Autodesk Inventor part; units mm, degrees
ref_plane "YZ Plane" through (0, 0, 0) normal (1, 0, 0) x (0, 1, 0)
ref_plane "XZ Plane" through (0, 0, 0) normal (0, 1, 0) x (-1, 0, 0)
ref_plane "XY Plane" through (0, 0, 0) normal (0, 0, 1) x (1, 0, 0)
sketch "Sketch1" plane through (0, 0, 0) normal (0, 0, 1) x (1, 0, 0)
  circle A0 centre (0, 0) radius 25.4
  dimension "d0" = 50.8
extrude "Extrusion1" add sketch "Sketch1" along normal blind 25.4 and the other way blind 101.6
sketch "Sketch2" plane through (0, 0, 0) normal (0, 1, 0) x (-1, 0, 0)
  line L0 (0, -25.4) -> (0, 152.4) construction
  line L1 (25.4, 25.4) -> (-25.4, 25.4) construction
  line L2 (0, 25.4) -> (-50.8, 25.4)
  line L3 (-50.8, 25.4) -> (-50.8, 127)
  line L4 (-50.8, 127) -> (0, 127)
  line L5 (0, 127) -> (0, 25.4)
  point P0 (0, 0)
  dimension "d8" = 50.8
  dimension "d9" = 101.6
revolve "Revolution1" add sketch "Sketch2" angle 360 about axis through (0, 0, -10) along (0, 0, 1)
sketch "Sketch3" plane through (0, 0, 0) normal (1, 0, 0) x (0, 1, 0)
  line L0 (50.8, 127) -> (-50.8, 127) construction
  line L1 (31.75, 127) -> (-31.75, 127)
  line L2 (-31.75, 127) -> (-31.75, 50.8)
  line L3 (-31.75, 50.8) -> (31.75, 50.8)
  line L4 (31.75, 50.8) -> (31.75, 127)
  line L5 (0, -25.4) -> (0, 152.4) construction
  point P0 (0, 0)
  point P1 (0, 50.8)
  dimension "d11" = 0
  dimension "d12" = 76.2
  dimension "d13" = 63.5
extrude "Extrusion2" cut sketch "Sketch3" along normal mid plane 254
sketch "Sketch4" plane through (0, 0, 0) normal (0, 1, 0) x (-1, 0, 0)
  line L0 (-39.6557, 127) -> (39.6557, 127) construction
  line L1 (39.6557, 127) -> (39.6557, 50.8) construction
  line L2 (-39.6557, 50.8) -> (-39.6557, 127) construction
  line L3 (-29.4957, 50.8) -> (-29.4957, 94.9643)
  line L4 (39.6557, 50.8) -> (-39.6557, 50.8) construction
  line L5 (29.4957, 94.9643) -> (29.4957, 50.8)
  arc A0 (29.4957, 94.9643) -> (-29.4957, 94.9643) centre (0, 94.9643) ccw
  line L6 (-29.4957, 50.8) -> (-112.68, 50.8)
  line L7 (-112.68, 50.8) -> (-112.68, 137.8838)
  line L8 (-112.68, 137.8838) -> (83.0957, 137.8838)
  line L9 (83.0957, 137.8838) -> (83.0957, 50.8)
  line L10 (83.0957, 50.8) -> (29.4957, 50.8)
  line L11 (39.6557, 127) -> (-39.6557, 127) construction
  point P0 (0, 0)
  point P1 (0, 124.46)
  point P2 (0, 127)
  point P3 (0, 127)
  dimension "d16" = 10.16
  dimension "d17" = 10.16
  dimension "d24" = 2.54
extrude "Extrusion3" cut sketch "Sketch4" along normal mid plane 254
sketch "Sketch5" plane through (0, 31.75, 94.9643) normal (0, -1, 0) x (1, 0, 0)
  circle A0 centre (0, 0) radius 15.875
  line L0 (29.4957, 0) -> (29.4957, -44.1643) construction
  line L1 (-29.4957, 0) -> (29.4957, 0) construction
  point P0 (0, -94.9643)
  dimension "d21" = 31.75
extrude "Extrusion4" add sketch "Sketch5" along normal up to next
properties part number "u_joint"
The listing builds one solid part. Answer for the finished solid, in the listing's coordinates (mm). A direction names the side the tool comes from. Give positions to 0.01 mm unless a question says otherwise; leave off trailing zeros. Write each loop counter-clockwise with the first axis right and the second up, starting at its lowest first coordinate (ties: lowest second). Pieces come first, ordered by that corner, then holes. Notation, with made-up numbers: (21.25, 13) -> (33.25, 13) arc R23 cw to (33.25, 45) -> close; hole circle Ø4 at (-34.75, -2.75). An arc over 180 degrees is marked (long way). Use a Markdown table: item, result.
(1) For faces 5 (the cylindrical face through (-5.506, -24.796, -37.211)), 6 (the flat face through (-7, -31.75, 80)), 7 (the flat face through (-29.496, 36, 73)), 8 (the flat face through (29.496, -37, 73)), determine the directions among +Z, -Z, +X, -X, +Y, -Y from which every point of the face is accessible in a straight line to the end or side of a thin tool.
Return value:
| item | result |
|---|---|
| face 5 | -Z |
| face 6 | none |
| face 7 | +Z, -X, +Y, -Y |
| face 8 | +Z, +X, +Y, -Y |
(2) Determine the mould class of faces 1 (the flat face through (10.6, 23.3, 25.4)), 2 (the cylindrical face through (0.649, -39.293, 124.453)), 3 (the flat face through (-29.496, -37, 73)), 4 (the cylindrical face through (-3.441, 0.444, 110.462)) for opening direction Z: released by +Z, released by -Z, zero draft, split by the parting line, or undercut.
Return value:
| item | result |
|---|---|
| face 1 | released by -Z |
| face 2 | released by +Z |
| face 3 | zero draft |
| face 4 | undercut |
(3) Section A-A, the plane y = 0 is taken. Determine the outline of the cut face in (x, z) (3 decimals).
Return value:
| item | result |
|---|---|
| outline | (-50.8, 25.4) -> (-25.4, 25.4) -> (-25.4, -101.6) -> (25.4, -101.6) -> (25.4, 25.4) -> (50.8, 25.4) -> (50.8, 50.8) -> (-50.8, 50.8) -> close; circle Ø31.75 at (0, 94.964) |
(4) Section C-C, the plane y = 35 is taken. Determine the outline of the cut face in (x, z), then the cut area to 3 significant figures.
Return value:
| item | result |
|---|---|
| outline | (-36.82, 25.4) -> (36.82, 25.4) -> (36.82, 50.8) -> (29.5, 50.8) -> (29.5, 94.96) arc R29.5 ccw to (-29.5, 94.96) -> (-29.5, 50.8) -> (-36.82, 50.8) -> close |
| area | 5,840 mm2 |
(5) Flat-ended cylindrical pins translate along their axes: P1, Ø12, axis at y = -1, z = 62, coming from the +X side; P2, Ø10.5, axis at y = -36.5, z = 72, coming from the +X side; P3, Ø2, axis at x = -12, z = 43, coming from the +Y side; P4, Ø12, axis at x = 29, z = -21.5, coming from the +Y side. Find the tip coordinate at first contact, or state that the pin passes through.
Return value:
| item | result |
|---|---|
| P1 | through |
| P2 | x = 29.5 |
| P3 | y = 49.59 |
| P4 | y = 10.78 |
(6) Section D-D, the plane z = -59.5 is taken. Determine the outline of the cut face in (x, y), then the cut area to 3 significant figures.
Return value:
| item | result |
|---|---|
| outline | circle Ø50.8 at (0, 0) |
| area | 2,030 mm2 |
(7) Find the intervals of material crossed by probe 1 along X at (y, z) = (29.5, 42); probe 2 along X at (y, z) = (1, -60.5); probe 3 along Z at (x, y) = (-33, 35), in increasing order. Write a range as from..to.
Return value:
| item | result |
|---|---|
| probe 1 | -41.36..41.36 |
| probe 2 | -25.38..25.38 |
| probe 3 | 25.4..50.8 |
(8) Section B-B, the plane x = 0 is taken. Determine the outline of the cut face in (y, z).
Return value:
| item | result |
|---|---|
| outline | (-50.8, 25.4) -> (-25.4, 25.4) -> (-25.4, -101.6) -> (25.4, -101.6) -> (25.4, 25.4) -> (50.8, 25.4) -> (50.8, 124.46) -> (31.75, 124.46) -> (31.75, 110.84) -> (-31.75, 110.84) -> (-31.75, 124.46) -> (-50.8, 124.46) -> close; hole (-31.75, 50.8) -> (31.75, 50.8) -> (31.75, 79.09) -> (-31.75, 79.09) -> close |
